Check sheet for the modelled part. Datum: model origin and axes. Units: mm. Give positions to 0.01 mm unless a question says otherwise; leave off trailing zeros. Order: outer loops, then holes, each group sorted by start corner. A loop starts at its lowest first (then second) coordinate and runs counter-clockwise, first axis right, second up. Notation, with made-up numbers: (12, 13.25) -> (20, 13.25) arc R12 cw to (20, 26.25) -> close; hole circle Ø11 at (19.25, 82.5). An arc over 180 degrees is marked (long way). One line per question, with ' | ' between items. Start each with the question number.
Autodesk Inventor part; units mm, degrees
ref_plane "YZ Plane" through (0, 0, 0) normal (1, 0, 0) x (0, 1, 0)
ref_plane "XZ Plane" through (0, 0, 0) normal (0, 1, 0) x (-1, 0, 0)
ref_plane "XY Plane" through (0, 0, 0) normal (0, 0, 1) x (1, 0, 0)
sketch "Sketch1" plane through (0, 0, 0) normal (0, 0, 1) x (1, 0, 0)
  line L0 (-140, -9) -> (140, -9)
  line L1 (140, -9) -> (140, 9)
  line L2 (140, 9) -> (-140, 9)
  line L3 (-140, 9) -> (-140, -9)
  line L4 (-140, -9) -> (140, 9) construction
  line L5 (140, -9) -> (-140, 9) construction
  point P0 (0, 0)
  dimension "d0" = 280
  dimension "d1" = 18
extrude "Extrusion1" add sketch "Sketch1" along normal blind 2
sketch "Sketch3" plane through (0, 0, 2) normal (0, 0, 1) x (1, 0, 0)
  line L0 (-99.5384, 1.5) -> (103.3668, 1.5) construction
  circle A0 centre (-70, 1.5) radius 2.25
  circle A1 centre (70, 1.5) radius 2.25
  line L1 (140, 9) -> (-140, 9)
  line L2 (-108, -2.5) -> (123, -2.5) construction
  line L3 (-140, -9) -> (140, -9)
  point P0 (0, 0)
  dimension "d4" = 4.5
  dimension "d5" = 4.5
  dimension "d6" = 7.5
  dimension "d7" = 6.5
  dimension "d8" = 70
  dimension "d9" = 70
extrude "Extrusion2" cut sketch "Sketch3" against normal blind 2
fillet "Fillet1" radius 2 4 edges at (-140, 9, 1) (-140, -9, 1) (140, 9, 1) (140, -9, 1)
sketch "Sketch4" plane through (0, 0, 2) normal (0, 0, 1) x (1, 0, 0)
  arc A0 (138, -9) -> (140, -7) centre (138, -7) ccw
  line L0 (140, -7) -> (140, 7)
  arc A1 (140, 7) -> (138, 9) centre (138, 7) ccw
  line L1 (138, 9) -> (-138, 9)
  arc A2 (-138, 9) -> (-140, 7) centre (-138, 7) ccw
  line L2 (-140, 7) -> (-140, -7)
  arc A3 (-140, -7) -> (-138, -9) centre (-138, -7) ccw
  line L3 (-138, -9) -> (138, -9)
  circle A4 centre (70, 1.5) radius 2.25
  circle A5 centre (-70, 1.5) radius 2.25
  point P0 (0, 0)
equation "\"d5\" = d4"
properties part number "DisplayAcrylicHolder"
1. Scan lines: probe 1 along X at (y, z) = (1, 0.7); probe 2 along Y at (x, z) = (-70, 1.65); probe 3 along X at (y, z) = (2.5, 1.3). Record each from-to range of solid material in increasing order.
2. Cross-section at B-B on y = 1.5. Record the boundary of the cut face in (x, z).
3. Cross-section at A-A on x = -70. Record the boundary of the cut face in (y, z).
4. Mould release check, pull along Y, two halves, no side actions. Record for faces 1 (the face through (-2, 0, 2)), 2 (the face through (72.08, 0.64, 1.01)): +Y half, -Y half, draft (parallel to the pull), parting line (faces both ways), or undercut.
5. Go/stop test with a flat-tipped pin: pin 1 (2.5 mm diameter, centred on x = -70, y = 1.5, fed in from +Z). Record where the tip stops, or that it passes through.
Response values:
1) probe 1: x = -140 to -72.19, -67.81 to 67.81, 72.19 to 140 | probe 2: y = -9 to -0.75, 3.75 to 9 | probe 3: x = -140 to -72.02, -67.98 to 67.98, 72.02 to 140
2) outline: (-140, 0) -> (-72.25, 0) -> (-72.25, 2) -> (-140, 2) -> close; (-67.75, 0) -> (67.75, 0) -> (67.75, 2) -> (-67.75, 2) -> close; (72.25, 0) -> (140, 0) -> (140, 2) -> (72.25, 2) -> close
3) outline: (-9, 0) -> (-0.75, 0) -> (-0.75, 2) -> (-9, 2) -> close; (3.75, 0) -> (9, 0) -> (9, 2) -> (3.75, 2) -> close
4) face 1: draft | face 2: undercut
5) pin 1: passes through
